from build123d import *

# Parameters (mm, degrees)
ESQUISSE1_W        = 150
ESQUISSE1_H        = 150
ESQUISSE1_R        = 22.5
BOSS_EXTRU_1_DEPTH = 10
CONG_1_R           = 22.5


with BuildPart() as part:
    # Esquisse1 → Boss.-Extru.1 (new body)
    with BuildSketch(Plane.XY):
        with Locations((75, 75)):
            Rectangle(ESQUISSE1_W, ESQUISSE1_H)
        with Locations((75, 75)):
            Circle(ESQUISSE1_R, mode=Mode.SUBTRACT)
    extrude(amount=BOSS_EXTRU_1_DEPTH)

    # Congé1
    cong_1_edges = [part.edges().sort_by_distance(p)[0] for p in [
        (0, 150, 5),
        (150, 150, 5),
        (150, 0, 5),
        (0, 0, 5),
    ]]
    fillet(cong_1_edges, radius=CONG_1_R)


solid = part.part
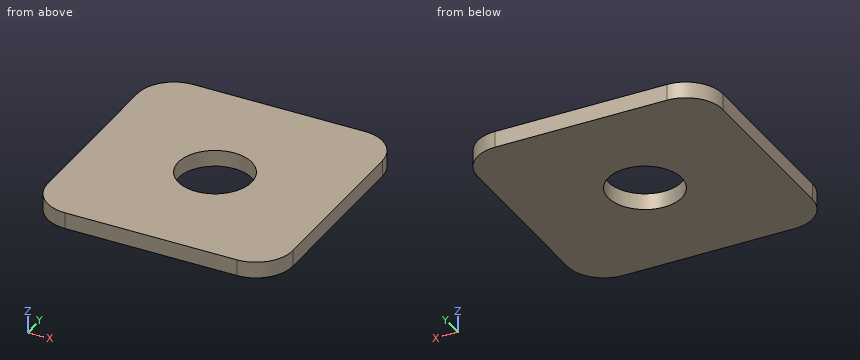
Geometry check sheet. Reference: the model listing, model coordinates, mm. Give positions to 0.01 mm unless a question says otherwise; leave off trailing zeros. Order: outer loops, then holes, each group sorted by start corner. A loop starts at its lowest first (then second) coordinate and runs counter-clockwise, first axis right, second up.
1) Cross-section at D-D (y = 11.5). Record the boundary of the cut face in (x, z), then the cut area to 3 significant figures.
Results are:
outline: (2.87, 0) - (147.13, 0) - (147.13, 10) - (2.87, 10) - close
area: 1,440 mm2
2) Gauge pin test, flat end, axial feed: pin 1 (5 mm diameter, centred on x = 51.5, y = 67.5, fed in from -Z). Record the tip position at first contact, or that the pin passes through.
Results are:
pin 1: stops at z = 0
3) Cross-section at A-A (y = 75). Record the boundary of the cut face in (x, z), then the cut area to 3 significant figures.
Results are:
outline: (0, 0) - (52.5, 0) - (52.5, 10) - (0, 10) - close; (97.5, 0) - (150, 0) - (150, 10) - (97.5, 10) - close
area: 1,050 mm2
4) Material ranges on probe 1 along X at (y, z) = (76, 9.25); probe 2 along Y at (x, z) = (75, 6.5); probe 3 along X at (y, z) = (73, 2.75), recorded low to high.
Results are:
probe 1: x = 0 to 52.52, 97.48 to 150
probe 2: y = 0 to 52.5, 97.5 to 150
probe 3: x = 0 to 52.59, 97.41 to 150
5) Cross-section at C-C (z = 4.25). Record the boundary of the cut face in (x, y), then the cut area to 3 significant figures.
Results are:
outline: (0, 22.5) arc R22.5 ccw to (22.5, 0) - (127.5, 0) arc R22.5 ccw to (150, 22.5) - (150, 127.5) arc R22.5 ccw to (127.5, 150) - (22.5, 150) arc R22.5 ccw to (0, 127.5) - close; hole circle Ø45 at (75, 75)
area: 20,500 mm2
